Geometry: final body of the model. Coordinates: model frame, mm. Round coordinates to 2 decimals unless told otherwise and drop trailing zeros. Write each loop counter-clockwise with the first axis right and the second up, starting at its lowest first coordinate (ties: lowest second). Pieces come first, ordered by that corner, then holes. Notation, with made-up numbers: M 76.25,52 L 122.25,52 A12 cw 122.25,74 Z; hole C 26.25,-6.5 d3. An arc over 180 degrees is marked long. Use one line per item in the form item = value. Start each with the question number.
Item 1: Section query D-D (y = 118). Return loops of the section in (x, z), and give its area (3 significant figures).
Item 2: Section query B-B (x = 59). Return loops of the section in (y, z).
Item 3: Section query A-A (z = 1.95). Return loops of the section in (x, y), and give its area (3 significant figures).
Item 4: Ray query, probe 1 along Y at (x, z) = (44.5, 2.15); probe 2 along Y at (x, z) = (66, 1.05); probe 3 along X at (y, z) = (103.5, 0.65). Return the intervals inside material, ascending.
Item 5: Pin query (flat end, axial travel): pin 1 Ø6 at (x, y) = (73.5, 36) entering from -Z; pin 2 Ø1.9 at (x, y) = (35.39, 10) entering from +Z; pin 3 Ø1 at (x, z) = (46, 0.5) entering from -Y. Return the tip coordinate at first contact, or that it passes through.
Item 6: Section query C-C (y = 136). Return loops of the section in (x, z).
from build123d import *

# Parameters (mm, degrees)
BOSS_EXTRUDE1_DEPTH = 3


with BuildPart() as part:
    # Sketch1 → Boss-Extrude1 (new body)
    with BuildSketch(Plane.XY):
        with BuildLine():
            ThreePointArc((33.820087007, 10.306516907), (31.717745776, 5.342686157), (31, 0))
            Line((31, 0), (37.5, 0))
            ThreePointArc((37.5, 0), (39.341287437, 6.871778265), (44.371778265, 11.902269093))
            ThreePointArc((44.371778265, 11.902269093), (88.737214743, 87.695526288), (46.196526291, 164.52780867))
            ThreePointArc((46.196526291, 164.52780867), (42.270857001, 165.080519331), (39.176809364, 162.60196377))
            Line((39.176809364, 162.60196377), (38.543843383, 161.408867573))
            ThreePointArc((38.543843383, 161.408867573), (39.597624954, 160.839941503), (40.643010869, 160.255731986))
            ThreePointArc((40.643010869, 160.255731986), (41.32681397, 162.784822546), (43.471778265, 161.280490828))
            ThreePointArc((43.471778265, 161.280490828), (42.902085601, 160.056372046), (41.598694773, 159.703967626))
            ThreePointArc((41.598694773, 159.703967626), (63.992298043, 140.41869644), (78.122959048, 114.462587877))
            ThreePointArc((78.122959048, 114.462587877), (79.754340696, 115.996827193), (81.321620809, 114.397161787))
            ThreePointArc((81.321620809, 114.397161787), (80.242557038, 112.884341426), (78.460839002, 113.41205812))
            ThreePointArc((78.460839002, 113.41205812), (82.110783268, 84.085055904), (75.158253764, 55.361241991))
            ThreePointArc((75.158253764, 55.361241991), (76.905197137, 55.720291583), (77.899174561, 54.239502389))
            ThreePointArc((77.899174561, 54.239502389), (76.240981534, 52.640560998), (74.703407596, 54.355811439))
            ThreePointArc((74.703407596, 54.355811439), (60.769047297, 33.338707308), (41.121778265, 17.531434218))
            ThreePointArc((41.121778265, 17.531434218), (37.422133199, 14.790870093), (34.437437632, 11.285209284))
            ThreePointArc((34.437437632, 11.285209284), (36.109888407, 11.429129733), (36.990452374, 10))
            ThreePointArc((36.990452374, 10), (35.236479303, 8.407425891), (33.820087007, 10.306516907))
        make_face()
    extrude(amount=BOSS_EXTRUDE1_DEPTH)


solid = part.part
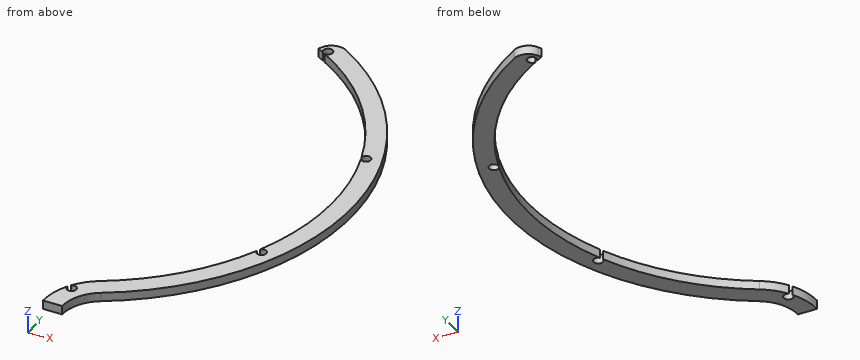
Working result:
q1.outline = M 76.87,0 L 83.79,0 L 83.79,3 L 76.87,3 Z
q1.area = 20.8 mm²
q2.outline = M 22.47,0 L 31.46,0 L 31.46,3 L 22.47,3 Z; M 146.05,0 L 155.05,0 L 155.05,3 L 146.05,3 Z
q3.outline = M 31,0 L 37.5,0 A13.74 cw 44.37,11.9 A88.74 ccw 46.2,164.53 A5 ccw 39.18,162.6 L 38.54,161.41 A82.24 cw 40.64,160.26 A1.6 cw long 41.6,159.7 A82.24 cw 78.12,114.46 A1.6 cw long 78.46,113.41 A82.24 cw 75.16,55.36 A1.6 cw long 74.7,54.36 A82.24 cw 41.12,17.53 A20.24 ccw 34.44,11.29 A1.6 cw long 33.82,10.31 A20.24 ccw Z
q3.area = 1,260 mm²
q4.probe_1 = 11.98 to 19.59, 157.92 to 165.18
q4.probe_2 = 29.43 to 39.69, 137.83 to 148.08
q4.probe_3 = 80.91 to 87.51
q5.pin_1 = 0
q5.pin_2 = through
q5.pin_3 = 12.56
q6.outline = M 67.32,0 L 75.12,0 L 75.12,3 L 67.32,3 Z
